Part print with two shaded views. Sizes in mm from the minimum x, y, z corner. A direction names the side the tool comes from. Round coordinates to 2 decimals unless told otherwise and drop trailing zeros. Write each loop counter-clockwise with the first axis right and the second up, starting at its lowest first coordinate (ties: lowest second). Pieces come first, ordered by that corner, then holes. Notation, with made-up numbers: M 85,1 L 136,1 A32 cw 136,34 Z; hole C -36,-36.75 d1. An arc over 180 degrees is marked long. One line per question, with ' | ' between items. Start each with the question number.
1) Saw through at D-D (z = 15). List the corners of the cut face in (x, y).
2) Drop flat-ended pins along their axis: pin 1 Ø1.9 at (x, y) = (5, 5) entering from -Z; pin 2 Ø5 at (y, z) = (4, 15.5) entering from -X; pin 3 Ø6 at (x, y) = (20, 3.5) entering from -Z. Give the stop position or say it passes through.
3) Saw through at B-B (y = 0.75). List the corners of the cut face in (x, z), plus the area to 3 significant figures.
4) Tool access for the marked faces 1, 2 and 3: list every direction of +Z, -Z, +X, -X, +Y, -Y with a clear straight run to the whole face (end or side of a thin tool).
5) Saw through at C-C (x = 23.5). List the corners of the cut face in (y, z).
6) Saw through at A-A (x = 5). List the corners of the cut face in (y, z), plus the area to 3 significant figures.
7) Wall check: probe 1 along X at (y, z) = (5, 1.85); probe 2 along Z at (x, y) = (3.75, 7.75). Give the ranges that are in metal, low to high. Write a range as [from, to].
8) Mould opens along Y. For the marked faces 4, 5 and 6 say: pulls with the +Y half, pulls with the -Y half, needs draft (parallel to the pull), parting line crosses it, or undercut.
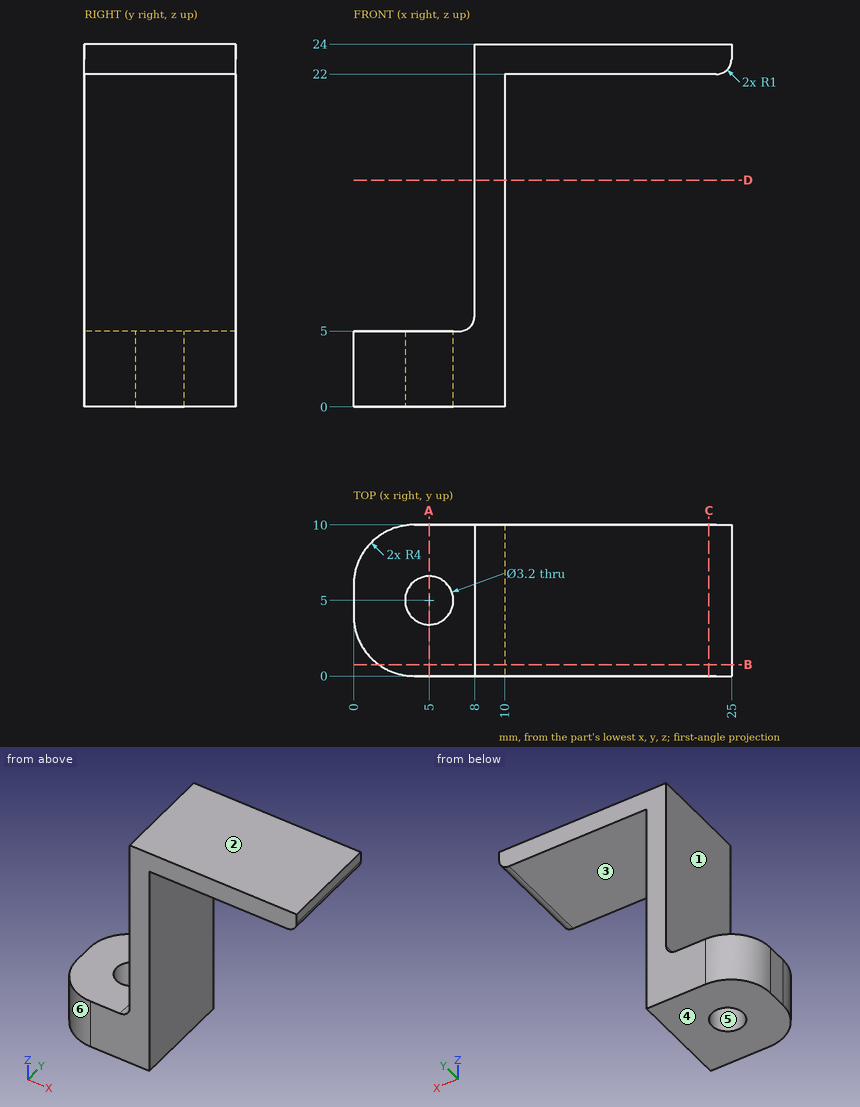
Answer key:
1) outline: M 8,0 L 10,0 L 10,10 L 8,10 Z
2) pin 1: passes through | pin 2: stops at x = 8 | pin 3: stops at z = 22
3) outline: M 1.67,0 L 10,0 L 10,22 L 24,22 A1 ccw 25,23 L 25,24 L 8,24 L 8,6 A1 cw 7,5 L 1.67,5 Z | area: 110 mm2
4) face 1: +Z, -X, +Y, -Y | face 2: +Z, +X, -X, +Y, -Y | face 3: -Z, +X, +Y, -Y
5) outline: M 0,22 L 10,22 L 10,24 L 0,24 Z
6) outline: M 0,0 L 3.4,0 L 3.4,5 L 0,5 Z; M 6.6,0 L 10,0 L 10,5 L 6.6,5 Z | area: 34.0 mm2
7) probe 1: x = [0, 3.4], [6.6, 10] | probe 2: z = [0, 5]
8) face 4: needs draft | face 5: undercut | face 6: pulls with the -Y half
